from build123d import *

# Parameters (mm, degrees)
F2_DEPTH        = 20
F2_COPIES_COUNT = 13
F4_DEPTH        = 20


# Not quite as in the source:
# - a pattern or mirror of a feature is missing from the dataset's text; its kind, count and spacing are read off the source's solid


with BuildPart() as f2:
    # F1 (on Front) → F2 (new body)
    with BuildSketch(Plane.XZ):
        with BuildLine():
            ThreePointArc((-14.0470065876, 104.0561464111), (0, 105), (14.0470065876, 104.0561464111))
            Line((14.0470065876, 104.0561464111), (16.7773367506, 121.0024649167))
            add(Edge.make_bspline(
                [(4.2468093523, 149.9398699824), (4.4290412164, 149.7210246606), (8.7826343305, 144.3294696938), (13.1358942294, 135.9586969958), (15.9340407786, 130.266903883), (16.7579313288, 121.3103558316), (16.7773367506, 121.0024649167)],
                knots=[0, 0, 0, 0, 0.2214991664, 0.5040555337, 0.7473622312, 1, 1, 1, 1], degree=3))
            ThreePointArc((4.2468093523, 149.9398699824), (0, 150), (-4.2468093523, 149.9398699824))
            add(Edge.make_bspline(
                [(-4.2468093523, 149.9398699824), (-4.4290412164, 149.7210246606), (-8.7826343305, 144.3294696938), (-13.1358942294, 135.9586969958), (-15.9340407786, 130.266903883), (-16.7579313288, 121.3103558316), (-16.7773367506, 121.0024649167)],
                knots=[0, 0, 0, 0, 0.2214991664, 0.5040555337, 0.7473622312, 1, 1, 1, 1], degree=3))
            Line((-16.7773367506, 121.0024649167), (-14.0470065876, 104.0561464111))
        make_face()
    extrude(amount=F2_DEPTH)


with BuildPart() as f2_copies_1:
    # F2_copies: instance of F2
    add(f2.part.rotate(Axis((0, 0, 0), (0, 1, 0)), 1 * 360 / F2_COPIES_COUNT))


with BuildPart() as f2_copies_2:
    # F2_copies: instance of F2
    add(f2.part.rotate(Axis((0, 0, 0), (0, 1, 0)), 2 * 360 / F2_COPIES_COUNT))


with BuildPart() as f2_copies_3:
    # F2_copies: instance of F2
    add(f2.part.rotate(Axis((0, 0, 0), (0, 1, 0)), 3 * 360 / F2_COPIES_COUNT))


with BuildPart() as f2_copies_4:
    # F2_copies: instance of F2
    add(f2.part.rotate(Axis((0, 0, 0), (0, 1, 0)), 4 * 360 / F2_COPIES_COUNT))


with BuildPart() as f2_copies_5:
    # F2_copies: instance of F2
    add(f2.part.rotate(Axis((0, 0, 0), (0, 1, 0)), 5 * 360 / F2_COPIES_COUNT))


with BuildPart() as f2_copies_6:
    # F2_copies: instance of F2
    add(f2.part.rotate(Axis((0, 0, 0), (0, 1, 0)), 6 * 360 / F2_COPIES_COUNT))


with BuildPart() as f2_copies_7:
    # F2_copies: instance of F2
    add(f2.part.rotate(Axis((0, 0, 0), (0, 1, 0)), 7 * 360 / F2_COPIES_COUNT))


with BuildPart() as f2_copies_8:
    # F2_copies: instance of F2
    add(f2.part.rotate(Axis((0, 0, 0), (0, 1, 0)), 8 * 360 / F2_COPIES_COUNT))


with BuildPart() as f2_copies_9:
    # F2_copies: instance of F2
    add(f2.part.rotate(Axis((0, 0, 0), (0, 1, 0)), 9 * 360 / F2_COPIES_COUNT))


with BuildPart() as f2_copies_10:
    # F2_copies: instance of F2
    add(f2.part.rotate(Axis((0, 0, 0), (0, 1, 0)), 10 * 360 / F2_COPIES_COUNT))


with BuildPart() as f2_copies_11:
    # F2_copies: instance of F2
    add(f2.part.rotate(Axis((0, 0, 0), (0, 1, 0)), 11 * 360 / F2_COPIES_COUNT))


with BuildPart() as f2_copies_12:
    # F2_copies: instance of F2
    add(f2.part.rotate(Axis((0, 0, 0), (0, 1, 0)), 12 * 360 / F2_COPIES_COUNT))


with BuildPart() as f2_1:
    add(f2.part)

    add(f2_copies_1.part)  # F4 merges F2_copies_1

    add(f2_copies_2.part)  # F4 merges F2_copies_2

    add(f2_copies_3.part)  # F4 merges F2_copies_3

    add(f2_copies_4.part)  # F4 merges F2_copies_4

    add(f2_copies_5.part)  # F4 merges F2_copies_5

    add(f2_copies_6.part)  # F4 merges F2_copies_6

    add(f2_copies_7.part)  # F4 merges F2_copies_7

    add(f2_copies_8.part)  # F4 merges F2_copies_8

    add(f2_copies_9.part)  # F4 merges F2_copies_9

    add(f2_copies_10.part)  # F4 merges F2_copies_10

    add(f2_copies_11.part)  # F4 merges F2_copies_11

    add(f2_copies_12.part)  # F4 merges F2_copies_12
    # F1 (on Front) → F4 (join)
    with BuildSketch(Plane.XZ):
        with BuildLine():
            ThreePointArc((-14.0470065876, 104.0561464111), (-69.1016074643, -79.0567381432), (105, 0))
            ThreePointArc((105, 0), (79.0567381432, 69.1016074643), (14.0470065876, 104.0561464111))
            ThreePointArc((14.0470065876, 104.0561464111), (0, 105), (-14.0470065876, 104.0561464111))
        make_face()
    extrude(amount=F4_DEPTH)


solid = f2_1.part
Geometry: final body of the model. Coordinates: model frame, mm. A direction names the side the tool comes from. Round coordinates to 2 decimals unless told otherwise and drop trailing zeros. Put each result on its own line as item: value. Start each with the question number.
(1) Material intervals for line 1 along Z through (x, y) = (107, -15.25); line 2 along X through (y, z) = (-17.75, 71); line 3 along X through (y, z) = (-6, -98), sorted ascending. Write a range as [from, to].
(2) Contact query for flat-ended pins moving along their axis: pin 1 Ø3 at (x, z) = (7.5, 29.5) entering from +Y; pin 2 Ø3 at (x, y) = (-6, -2) entering from -Z; pin 3 Ø8 at (x, y) = (73, -3.5) entering from +Z; pin 4 Ø12 at (x, y) = (-0.5, -13.5) entering from +Z. Output: stop coordinate, or through.
(3) Draft query along X for faces 1 (the face through (-148.9, -9.86, 18.14)), 2 (the face through (110.8, -9.86, -25.517)), 3 (the face through (-113.69, -9.86, -1.74)). Return one class per face: +X half, -X half, draft (parallel to the pull), parting line (faces both ways), or undercut.
(4) Set-up query: faces 4 (the face through (101.26, -9.86, 51.19)), 5 (the face through (38.686, -9.86, 106.916)), 6 (the face through (99.647, -9.86, -54.254)). Return all of +Z, -Z, +X, -X, +Y, -Y with unobstructed straight access to the full face (end or side cutting, diameter ignored); none if empty.
Findings below:
1. line 1: z = [-58.49, -24.74], [-1.48, 28.04], [53.92, 88.35]
1. line 2: x = [-121.71, -78], [-77.36, 77.36], [78, 121.71]
1. line 3: x = [-101.16, -65.34], [-38.68, 38.68], [65.34, 101.16]
2. pin 1: stops at y = 0
2. pin 2: stops at z = -104.9
2. pin 3: stops at z = 133.19
2. pin 4: stops at z = 150
3. face 1: -X half
3. face 2: +X half
3. face 3: undercut
4. face 4: +X, +Y, -Y
4. face 5: +Z, +Y, -Y
4. face 6: +Y, -Y
